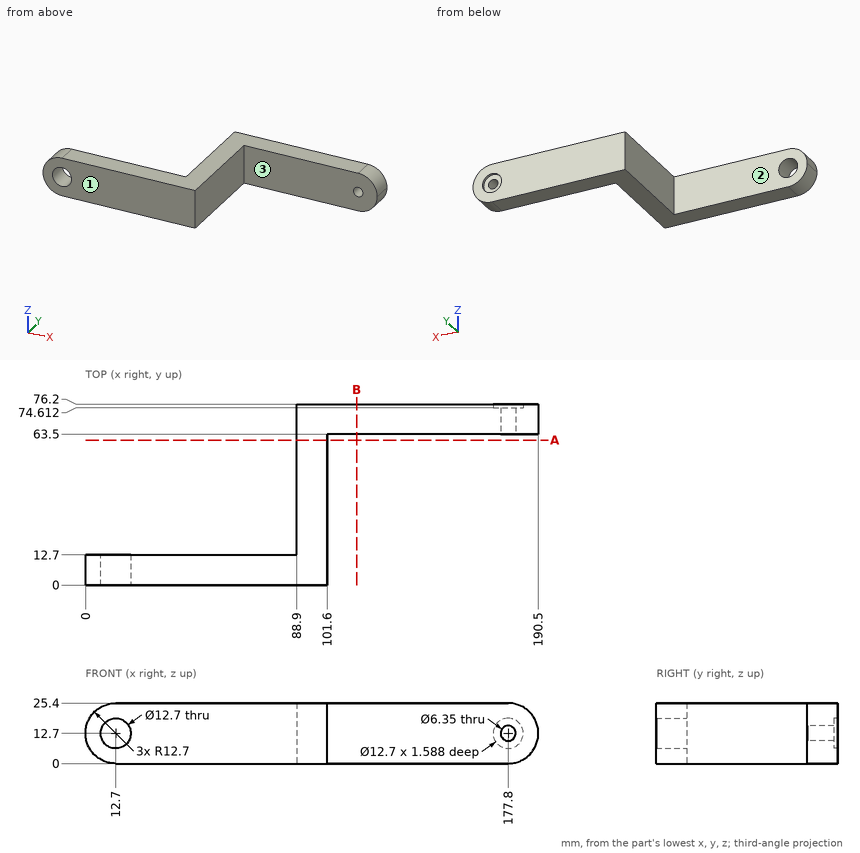
For this review, use the dimensioned drawing (mm, ordinates from the lowest corner) and the shaded views. A direction names the side the tool comes from. Give positions to 0.01 mm unless a question says otherwise; leave off trailing zeros. Order: outer loops, then holes, each group sorted by start corner. A loop starts at its lowest first (then second) coordinate and runs counter-clockwise, first axis right, second up. Notation, with made-up numbers: (21, 82) -> (30, 82) arc R18 cw to (30, 93) -> close; hole circle Ø3 at (47.25, 37.5). An arc over 180 degrees is marked (long way). Write item = value, one per line. Start each with the question number.
(1) Take a section at B-B (x = 114). Write out the cut boundary in (y, z), plus the area to 3 significant figures.
(2) Tool access review of the marked faces 1, 2 and 3: name each direction out of +Z, -Z, +X, -X, +Y, -Y from which nothing blocks a thin tool from reaching the whole face with its end or side.
(3) For pin 1 Ø12 at (x, z) = (127, 20.5) entering from -Y; pin 2 Ø12 at (y, z) = (26.5, 6) entering from +X; pin 3 Ø7.5 at (x, z) = (177.8, 12.7) entering from +Y, all flat-tipped, find the tip position at first contact; note any pin that passes through.
(4) Take a section at A-A (y = 61). Write out the cut boundary in (x, z), plus the area to 3 significant figures.
(5) For L1, parallel to X at y = 69.5, z = 12.7 (1 decimal); L2, parallel to Z at x = 177.8, y = 75.4; L3, parallel to X at y = 9.75, z = 12.7, list the stretches that pass through material, from the lowest coordinate up. Write a range as from..to.
Returned:
q1.outline = (63.5, 0) -> (76.2, 0) -> (76.2, 25.4) -> (63.5, 25.4) -> close
q1.area = 323 mm²
q2.face_1 = +Z, -Z, +X, -X, -Y
q2.face_2 = +Z, -Z, -X, +Y
q2.face_3 = +Z, -Z, +X, -Y
q3.pin_1 = 63.5
q3.pin_2 = 101.6
q3.pin_3 = 74.61
q4.outline = (88.9, 0) -> (101.6, 0) -> (101.6, 25.4) -> (88.9, 25.4) -> close
q4.area = 323 mm²
q5.L1 = 88.9..174.6, 181..190.5
q5.L2 = 0..6.35, 19.05..25.4
q5.L3 = 0..6.35, 19.05..101.6
